Design review of the part built by this model. Coordinates are the model's own, in mm. Face numbers are marked on the shaded views. Give positions to 0.01 mm unless a question says otherwise; leave off trailing zeros. Order: outer loops, then holes, each group sorted by start corner. A loop starts at its lowest first (then second) coordinate and runs counter-clockwise, first axis right, second up.
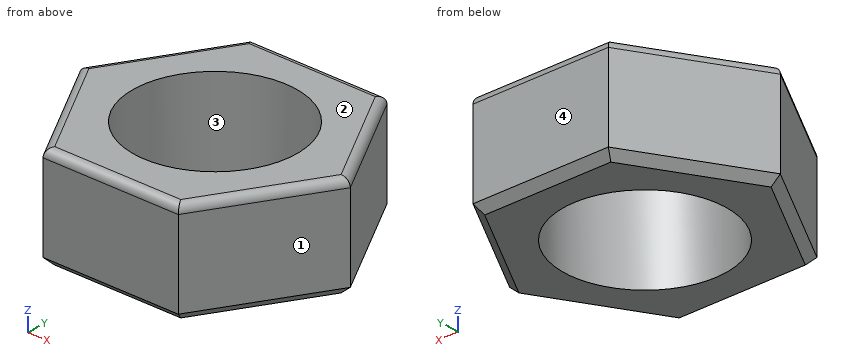
```python
from build123d import *

# Parameters (mm, degrees)
F1_DEPTH = 6.3
F3_R     = 0.5
F4_D     = 10
F5_SIZE  = 0.5


with BuildPart() as f1:
    # F0 (on Top) → F1 (new body)
    with BuildSketch(Plane.XY):
        Polygon((4.25, -7.361216), (8.5, 0), (4.25, 7.361216), (-4.25, 7.361216), (-8.5, 0), (-4.25, -7.361216), align=None)
    extrude(amount=F1_DEPTH)

    # F3
    f3_edges = [f1.edges().sort_by_distance(p)[0] for p in [
        (0, -7.361216, 6.3),
        (6.375, -3.680608, 6.3),
        (6.375, 3.680608, 6.3),
        (0, 7.361216, 6.3),
        (-6.375, 3.680608, 6.3),
        (-6.375, -3.680608, 6.3),
    ]]
    fillet(f3_edges, radius=F3_R)

    # F4 (through all)
    with Locations(Plane(origin=(0, 0, 0), x_dir=(1, 0, 0), z_dir=(0, 0, -1))):
        with Locations((0, 0)):
            Hole(F4_D / 2)

    # F5
    f5_edges = [f1.edges().sort_by_distance(p)[0] for p in [
        (-6.375, 3.680608, 0),
        (0, 7.361216, 0),
        (-6.375, -3.680608, 0),
        (0, -7.361216, 0),
        (6.375, -3.680608, 0),
        (6.375, 3.680608, 0),
    ]]
    chamfer(f5_edges, length=F5_SIZE)


solid = f1.part
```
1. Take a section at C-C (x = -2.75). State the section outline as (y, z) points.
Recorded:
outline: (-7.36, 0.5) - (-6.86, 0) - (-4.18, 0) - (-4.18, 6.3) - (-6.86, 6.3) arc R0.5 ccw to (-7.36, 5.8) - close; (4.18, 0) - (6.86, 0) - (7.36, 0.5) - (7.36, 5.8) arc R0.5 ccw to (6.86, 6.3) - (4.18, 6.3) - close
2. Take a section at A-A (x = 0). State the section outline as (y, z) points.
Recorded:
outline: (-7.36, 0.5) - (-6.86, 0) - (-5, 0) - (-5, 6.3) - (-6.86, 6.3) arc R0.5 ccw to (-7.36, 5.8) - close; (5, 0) - (6.86, 0) - (7.36, 0.5) - (7.36, 5.8) arc R0.5 ccw to (6.86, 6.3) - (5, 6.3) - close
3. Take a section at B-B (z = 2.75). State the section outline as (x, y) points.
Recorded:
outline: (-8.5, 0) - (-4.25, -7.36) - (4.25, -7.36) - (8.5, 0) - (4.25, 7.36) - (-4.25, 7.36) - close; hole circle Ø10 at (0, 0)
4. For line 1 along Y through (x, z) = (0, 5.25); line 2 along X through (y, z) = (1, 2.75); line 3 along X through (y, z) = (-1.75, 0.75), list the stretches that pass through material, from the lowest coordinate up.
Recorded:
line 1: y = -7.36 to -5, 5 to 7.36
line 2: x = -7.92 to -4.9, 4.9 to 7.92
line 3: x = -7.49 to -4.68, 4.68 to 7.49
5. For pin 1 (1 mm diameter, centred on x = 5.5, z = 1.5, fed in from +Y); pin 2 (6 mm diameter, centred on x = 0, y = 0, fed in from +Z); pin 3 (8 mm diameter, centred on x = -4, y = -2.5, fed in from +Z); pin 4 (3 mm diameter, centred on y = 5, z = 5.5, fed in from +X), all flat-tipped, find the tip position at first contact; note any pin that passes through.
Recorded:
pin 1: stops at y = 6.06
pin 2: passes through
pin 3: stops at z = 6.3
pin 4: stops at x = 6.48
6. Draft analysis for pull direction Y (two halves, no side actions). For the marked faces 1, 2, 3 and 4, state which applies: pulls with the +Y half, pulls with the -Y half, needs draft (parallel to the pull), parting line crosses it, or undercut.
Recorded:
face 1: pulls with the -Y half
face 2: needs draft
face 3: undercut
face 4: pulls with the +Y half
